```python
from build123d import *


with BuildPart() as f2:
    # F0 (on Top) → F2 section 0
    with BuildSketch(Plane.XY, mode=Mode.PRIVATE) as f2_s0:
        Polygon((12.7, -17.48005039), (20.5490316571, 6.6767851239), (0, 21.6065305321), (-20.5490316571, 6.6767851239), (-12.7, -17.48005039), align=None)
    loft([f2_s0.sketch, Vertex(0, 0, 19.05)])

    # F0 (on Top) → F3 section 0
    with BuildSketch(Plane.XY, mode=Mode.PRIVATE) as f3_s0:
        Polygon((12.7, -17.48005039), (20.5490316571, 6.6767851239), (0, 21.6065305321), (-20.5490316571, 6.6767851239), (-12.7, -17.48005039), align=None)
    loft([f3_s0.sketch, Vertex(0, 0, -19.05)])


solid = f2.part
```
Geometry check sheet. Reference: the model listing, model coordinates, mm. Give positions to 0.01 mm unless a question says otherwise; leave off trailing zeros. Order: outer loops, then holes, each group sorted by start corner. A loop starts at its lowest first (then second) coordinate and runs counter-clockwise, first axis right, second up. Notation, with made-up numbers: (34, -38) - (92, -38) arc R19 cw to (92, -2) - close; hole circle Ø7 at (-27.75, 24.25). An arc over 180 degrees is marked (long way). Write item = value, one per line. Start each with the question number.
1) Section check A-A (x = -2). Enter the section's corners in (y, z), then the cut area to 3 significant figures.
2) Gauge pin test, flat ends, axial feed: pin 1 Ø4 at (y, z) = (-12.5, 4) entering from -X (3 decimals); pin 2 Ø10 at (y, z) = (-10, -4.5) entering from +X; pin 3 Ø5 at (y, z) = (-9, 10.5) entering from -X; pin 4 Ø6 at (x, y) = (-0.5, 1.5) entering from -Z. Record the tip position at first contact, or that the pin passes through.
3) Section check D-D (z = 14). Enter the section's corners in (x, y), then the cut area to 3 significant figures.
4) Section check C-C (z = -11). Enter the section's corners in (x, y), then the cut area to 3 significant figures.
5) Scan lines: L1, parallel to Z at x = 6, y = 2.5; L2, parallel to Z at x = 16, y = 9; L3, parallel to X at y = 1, z = -7.5. Record each from-to range of solid material in increasing order.
6) Section check B-B (y = -10). Enter the section's corners in (x, z), then the cut area to 3 significant figures.
7) Draft check along X on faces 1 (the flat face through (-0.2, -10.6, -7.5)), 2 (the flat face through (6.35, 8.44, 7.54)), 3 (the flat face through (-10.1, -3.09, 7.54)). Enter one of: released by +X, released by -X, zero draft, split by the parting line, or undercut.
Geometry check:
q1.outline = (-17.48, 0) - (-2.75, -16.05) - (0.65, -17.2) - (20.15, 0) - (0.65, 17.2) - (-2.75, 16.05) - close
q1.area = 685 mm2
q2.pin_1 = -12.495
q2.pin_2 = 15.84
q2.pin_3 = -7.87
q2.pin_4 = -19.05
q3.outline = (-5.45, 1.77) - (-3.37, -4.63) - (3.37, -4.63) - (5.45, 1.77) - (0, 5.73) - close
q3.area = 78.0 mm2
q4.outline = (-8.68, 2.82) - (-5.37, -7.39) - (5.37, -7.39) - (8.68, 2.82) - (0, 9.13) - close
q4.area = 198 mm2
q5.L1 = -13 to 13
q5.L2 = -0.87 to 0.87
q5.L3 = -11.47 to 11.47
q6.outline = (-15.13, 0) - (-7.27, -8.15) - (7.27, -8.15) - (15.13, 0) - (7.27, 8.15) - (-7.27, 8.15) - close
q6.area = 365 mm2
q7.face_1 = zero draft
q7.face_2 = released by +X
q7.face_3 = released by -X
